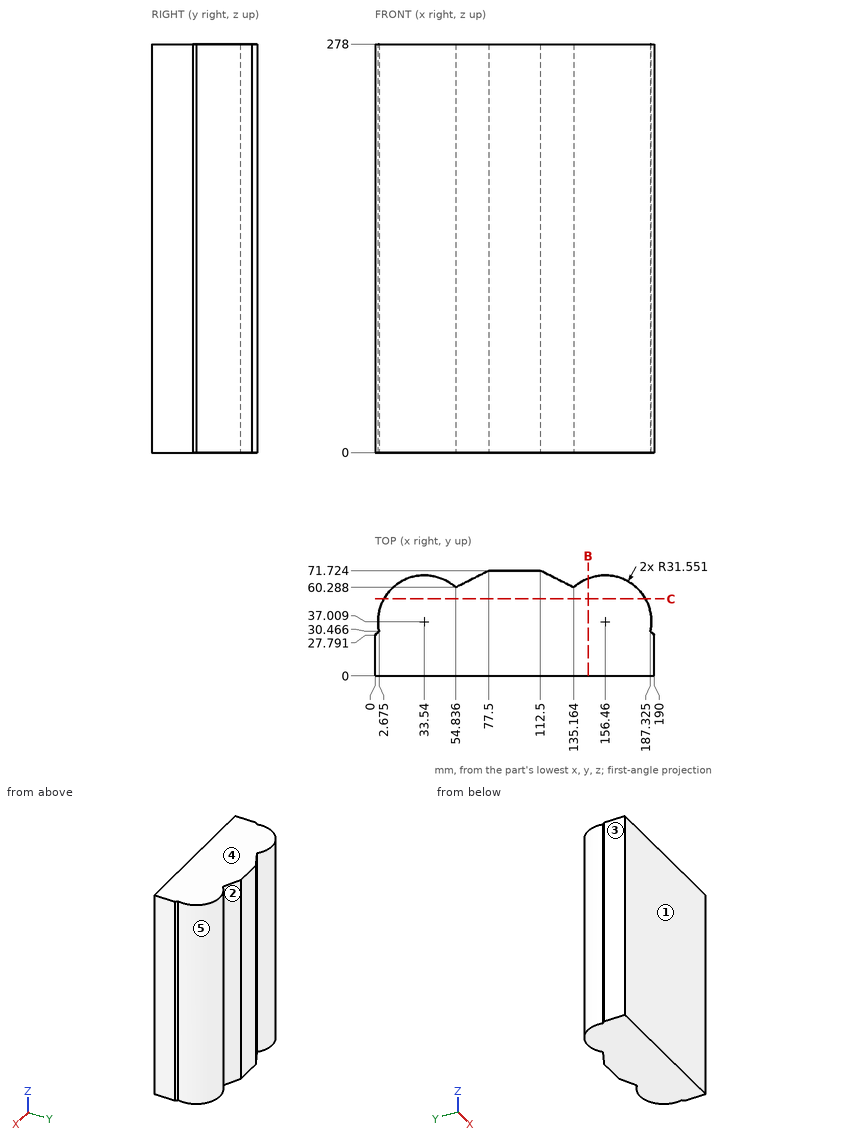
Geometry check sheet. Reference: drawing and pictorial views, mm from the part's lowest x, y, z. A direction names the side the tool comes from. Round coordinates to 2 decimals unless told otherwise and drop trailing zeros. Order: outer loops, then holes, each group sorted by start corner. A loop starts at its lowest first (then second) coordinate and runs counter-clockwise, first axis right, second up. Notation, with made-up numbers: (54.25, 88.5) -> (95.25, 88.5) arc R24 cw to (95.25, 124.5) -> close; hole circle Ø4 at (52, -28.75). An arc over 180 degrees is marked (long way). One line per item, written item: value. Start each with the question number.
Q1. Cross-section at B-B (x = 145). Record the boundary of the cut face in (y, z) (1 decimal), and give its area (3 significant figures).
Q2. Thickness scan on line 1 (X direction, y = 64.5, z = 236) (1 decimal); line 2 (X direction, y = 39, z = 103.5); line 3 (Y direction, x = 128, z = 110) (1 decimal). Record the ranges inside material, lowest first.
Q3. Mould release check, pull along X, two halves, no side actions. Record for the marked faces 3, 4 and 5: pulls with the +X half, pulls with the -X half, needs draft (parallel to the pull), parting line crosses it, or undercut.
Q4. Gauge pin test, flat ends, axial feed: pin 1 Ø5 at (y, z) = (61, 218) entering from +X; pin 2 Ø1.5 at (y, z) = (63.5, 71) entering from -X (1 decimal); pin 3 Ø12 at (x, z) = (132.5, 53) entering from +Y. Record the tip position at first contact, or that the pin passes through.
Q5. Set-up check for the marked faces 1 and 2: record each of +Z, -Z, +X, -X, +Y, -Y from which the full face is reachable in a straight line by a thin tool's end or side.
Q6. Cross-section at C-C (y = 52.5). Record the boundary of the cut face in (x, z), and give its area (3 significant figures).
Completed:
1. outline: (0, 0) -> (66.4, 0) -> (66.4, 278) -> (0, 278) -> close
1. area: 18,500 mm²
2. line 1: x = 18.1 to 49, 63.2 to 126.8, 141 to 171.9
2. line 2: x = 2.05 to 187.95
2. line 3: y = 0 to 63.9
3. face 3: pulls with the -X half
3. face 4: needs draft
3. face 5: undercut
4. pin 1: stops at x = 179.56
4. pin 2: stops at x = 15.3
4. pin 3: stops at y = 64.66
5. face 1: +Z, -Z, +X, -X, -Y
5. face 2: +Z, -Z, +Y
6. outline: (6.05, 0) -> (183.95, 0) -> (183.95, 278) -> (6.05, 278) -> close
6. area: 49,500 mm²
